Autodesk Fusion 360 part; units mm, degrees
sketch "Sketch1" plane through (0, 0, 0) normal (0, 1, 0) x (1, 0, 0)
  line L0 (-4, 12.7291) -> (-4, 24.6266)
  line L1 (0, 24.6266) -> (0, 12.7291)
  line L2 (-1.1892, 37.3052) -> (1, 42)
  line L3 (2.436, 35.6147) -> (2.4713, 35.6905)
  line L4 (35, 38) -> (6.0966, 38)
  line L5 (1, 6.3908) -> (1, 42)
  line L6 (1, 42) -> (35, 42)
  line L7 (35, 42) -> (35, 38)
  arc A0 (-1.1892, 37.3052) -> (-4, 24.6266) centre (26, 24.6266) ccw
  arc A1 (2.436, 35.6147) -> (0, 24.6266) centre (26, 24.6266) ccw
  arc A2 (6.0966, 38) -> (2.4713, 35.6905) centre (6.0966, 34) ccw
  line L8 (0, 12.7291) -> (0, 0)
  line L9 (0, 0) -> (-4, 0)
  line L10 (-4, 0) -> (-4, 12.7291)
  line L11 (-2.8767, 0) -> (-2.8767, -1.8)
  line L12 (-2.8767, 0) -> (-2.8767, 1.8)
  line L13 (-2.8767, -1.8) -> (-1.3767, 0)
  line L14 (-2.8767, 1.8) -> (-1.3767, 0)
  line L15 (-2.8767, 1.8) -> (-4.3767, 0)
  line L16 (-2.8767, -1.8) -> (-4.3767, 0)
  line L17 (-2.8767, -1.6438) -> (-4.2999, 0.064)
  line L18 (-2.8767, -1.6438) -> (-1.4535, 0.064)
  line L19 (-4, 0) -> (-6, 0)
  line L20 (-6, 0) -> (-6, 2.7)
  line L21 (-4, 1.5) -> (-4, 0)
  line L22 (-5.5915, 4.0695) -> (-4, 6.5)
  arc A3 (-5.5915, 4.0695) -> (-6, 2.7) centre (-3.5, 2.7) ccw
  line L23 (-1.3827, 0) -> (-4.3827, 0)
  line L24 (-4.3827, 0) -> (-1.3636, 0) construction
  line L25 (-3.8767, 0) -> (-1.8767, 0)
  line L26 (-1.8767, 0) -> (-1.8767, 3)
  line L27 (-1.8767, 3) -> (-3.8767, 3)
  line L28 (-3.8767, 3) -> (-3.8767, 0)
  line L29 (-1.8767, 3) -> (-1.9572, 0.6965)
  line L30 (-1.8767, 3) -> (0.4282, 3) construction
  line L31 (-3.8767, 3) -> (-3.7963, 0.6965)
  dimension "d5" = 4
  dimension "d6" = 30
  dimension "d7" = 26
  dimension "d8" = 4
  dimension "d9" = 1.8
  dimension "d10" = 1.8
  dimension "d11" = 1.5
  dimension "d12" = 1.5
  dimension "d13" = 0.1
  dimension "d30" = 4
  dimension "d33" = 4
  dimension "d36" = 5
  dimension "d38" = 35
  dimension "d60" = 25
  dimension "d113" = 2
  dimension "d115" = 2.5
  dimension "d126" = 6.5
  dimension "d334" = 4
  dimension "d335" = 38
  dimension "d486" = 1
  dimension "d487" = 1
  dimension "d488" = 3
  dimension "d489" = 2.8767
  dimension "d490" = 92
  dimension "d491" = 88
sketch "Sketch2" plane through (0, 0, 0) normal (0, 0, 1) x (1, 0, 0)
  line L0 (15, 70) -> (55, 70)
  line L1 (70, 55) -> (70, -55)
  line L2 (55, -70) -> (15, -70)
  line L3 (0, -55) -> (0, 55)
  arc A0 (15, 70) -> (0, 55) centre (15, 55) ccw
  arc A1 (70, 55) -> (55, 70) centre (55, 55) ccw
  arc A2 (55, -70) -> (70, -55) centre (55, -55) ccw
  arc A3 (0, -55) -> (15, -70) centre (15, -55) ccw
  dimension "d14" = 15
  dimension "d15" = 15
  dimension "d16" = 15
  dimension "d17" = 15
  dimension "d39" = 70
  dimension "d40" = 140
sketch "Sketch24" plane through (0, 0, 0) normal (0, 1, 0) x (1, 0, 0)
  line L0 (-1.8767, 3) -> (-3.8767, 3)
  line L1 (-3.7967, 3) -> (-3.6989, 0.2)
  line L2 (-4.3827, 0) -> (-1.3636, 0)
  line L3 (-3.6989, 0.2) -> (-2.0546, 0.2)
  line L4 (-2.0546, 0.2) -> (-1.9568, 3)
  line L5 (-1.9568, 3) -> (-3.7967, 3)
  line L6 (-3.8767, 3) -> (-3.7963, 0.6965)
  line L7 (-1.8767, 3) -> (-1.9572, 0.6965)
  arc A0 (-3.6989, 0.2) -> (-2.0546, 0.2) centre (-2.8767, 1.7053) ccw
  dimension "d493" = 0.08
  dimension "d494" = 0.08
  dimension "d495" = 2.8
  dimension "d538" = 1.7152
sweep "Sweep4" add profiles "Sketch24" path "Sketch2" along A0 L0 A1 L1 A2 L2 A3 L3 section 1
equation "d5 = Twall"
equation "d6 = Rbase"
equation "d7 = Rbase - Twall"
equation "d14 = Rcorner"
equation "d15 = Rcorner"
equation "d16 = Rcorner"
equation "d17 = Rcorner"
equation "Twall = 4 mm"
equation "length = 140 mm"
equation "width = 70 mm"
equation "height = 38 mm"
equation "Rcorner = 15 mm"
equation "Rbase = 30 mm"
equation "d30 = Twall"
equation "d33 = Twall"
equation "d36 = base_inset"
equation "base_inset = 5 mm"
equation "d38 = width * 0.5"
equation "d39 = width"
equation "d40 = length"
equation "d60 = base_ang"
equation "base_ang = 25 deg"
equation "d334 = Twall"
equation "d335 = height"
equation "d495 = oringHeight"
equation "oringHeight = 2.8 mm"
The model under review builds one solid part; all positions refer to its coordinate system, in mm. A direction names the side the tool comes from. Round coordinates to 2 decimals unless told otherwise and drop trailing zeros. Loops run counter-clockwise (first coordinate to the right, second up) from the corner with the lowest first, then second, coordinate; pieces in that order, holes last. Notation, with made-up numbers: M 56.5,25 L 94.5,25 A17 cw 94.5,41 Z; hole C -26.75,23.5 d11. An arc over 180 degrees is marked long. Answer as a JSON object with one key per item and string values.
Item 1: We need section A-A, the plane y = -33. State the section outline as (x, z) points, and give its area (3 significant figures).
Check sheet entries:
{"outline": "M -3.8,-3 L -1.96,-3 L -2.05,-0.2 A1.72 ccw -3.7,-0.2 Z; M 71.96,-3 L 73.8,-3 L 73.7,-0.2 A1.72 ccw 72.05,-0.2 Z", "area": "10.2 mm2"}
Item 2: We need section B-B, the plane x = 28.5. State the section outline as (y, z) points, and give its area (3 significant figures).
Check sheet entries:
{"outline": "M -73.8,-3 L -71.96,-3 L -72.05,-0.2 A1.72 ccw -73.7,-0.2 Z; M 71.96,-3 L 73.8,-3 L 73.7,-0.2 A1.72 ccw 72.05,-0.2 Z", "area": "10.2 mm2"}
Item 3: We need section C-C, the plane z = -2. State the section outline as (x, y) points.
Check sheet entries:
{"outline": "M -3.76,-55 A18.76 ccw 15,-73.76 L 55,-73.76 A18.76 ccw 73.76,-55 L 73.76,55 A18.76 ccw 55,73.76 L 15,73.76 A18.76 ccw -3.76,55 Z; hole M -1.99,-55 A16.99 ccw 15,-71.99 L 55,-71.99 A16.99 ccw 71.99,-55 L 71.99,55 A16.99 ccw 55,71.99 L 15,71.99 A16.99 ccw -1.99,55 Z"}
Item 4: For line 1 along Y through (x, z) = (35, -2.75); line 2 along X through (y, z) = (56, -1.6); line 3 along Y through (x, z) = (25, -0.7), list the stretches that pass through material, from the lowest coordinate up.
Check sheet entries:
{"line 1": "-73.79 to -71.97, 71.97 to 73.79", "line 2": "-3.72 to -1.98, 71.98 to 73.72", "line 3": "-73.72 to -72.04, 72.04 to 73.72"}
Item 5: The part is to be moulded in two halves that separate along Y. For faces 3 (the face through (68.11, 68.4, -1.62)), 4 (the face through (73, 0, -3)), 5 (the face through (3.11, 67.16, -1.58)), 6 (the face through (66.89, -67.16, -1.58)), say which applies: +Y half, -Y half, draft (parallel to the pull), parting line (faces both ways), or undercut.
Check sheet entries:
{"face 3": "+Y half", "face 4": "draft", "face 5": "undercut", "face 6": "undercut"}
Item 6: Tool access review of faces 1 (the face through (1.6, 68.11, -1.62)), 2 (the face through (67.16, 66.89, -1.58)): name each direction out of +Z, -Z, +X, -X, +Y, -Y from which nothing blocks a thin tool from reaching the whole face with its end or side.
Check sheet entries:
{"face 1": "+Z, -X, +Y", "face 2": "+Z"}
